```python
from build123d import *

# Parameters (mm, degrees)
SZKIC1_W                       = 90
SZKIC1_H                       = 62
DODANIE_WYCI_GNI_CIE1_DEPTH    = 12
OTW_R_GWINTOWANY_M5X0_81_D     = 4.2
OTW_R_GWINTOWANY_M5X0_81_DEPTH = 14
OTW_R_GWINTOWANY_M5X0_81_TIP   = 1.2618073
OTW_R_GWINTOWANY_M5X0_82_D     = 4.2
OTW_R_GWINTOWANY_M5X0_82_DEPTH = 20
OTW_R_GWINTOWANY_M5X0_82_TIP   = 1.2618073


with BuildPart() as part:
    # Szkic1 → Dodanie-wyciągnięcie1 (new body)
    with BuildSketch(Plane.XY):
        with Locations((73, 300)):
            Rectangle(SZKIC1_W, SZKIC1_H)
    extrude(amount=DODANIE_WYCI_GNI_CIE1_DEPTH)

    # Otwór gwintowany M5x0.81
    with Locations(Plane.XY.offset(12)):
        with Locations((97, 323), (79, 323), (79, 277), (97, 277)):
            Hole(OTW_R_GWINTOWANY_M5X0_81_D / 2, depth=OTW_R_GWINTOWANY_M5X0_81_DEPTH)
            with Locations((0, 0, -(OTW_R_GWINTOWANY_M5X0_81_DEPTH + OTW_R_GWINTOWANY_M5X0_81_TIP / 2))):  # 118° drill point
                Cone(0, OTW_R_GWINTOWANY_M5X0_81_D / 2, OTW_R_GWINTOWANY_M5X0_81_TIP, mode=Mode.SUBTRACT)

    # Otwór gwintowany M5x0.82
    with Locations(Plane.ZY.offset(-28)):
        with Locations((6, 286), (6, 314)):
            Hole(OTW_R_GWINTOWANY_M5X0_82_D / 2, depth=OTW_R_GWINTOWANY_M5X0_82_DEPTH)
            with Locations((0, 0, -(OTW_R_GWINTOWANY_M5X0_82_DEPTH + OTW_R_GWINTOWANY_M5X0_82_TIP / 2))):  # 118° drill point
                Cone(0, OTW_R_GWINTOWANY_M5X0_82_D / 2, OTW_R_GWINTOWANY_M5X0_82_TIP, mode=Mode.SUBTRACT)


solid = part.part
```
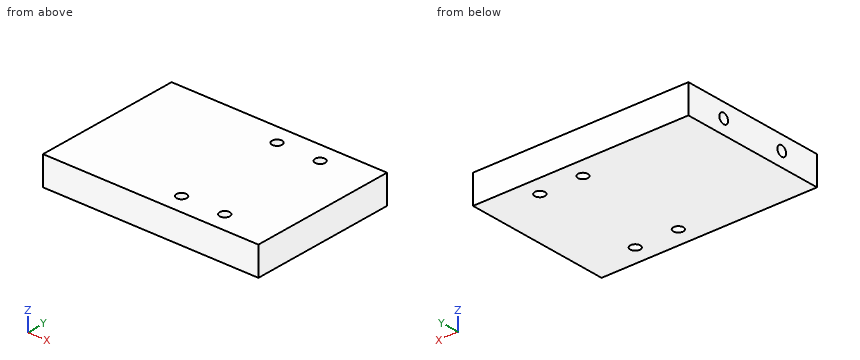
Could you check a few things on this model? Use its own coordinates, in mm. Give positions to 0.01 mm unless a question says otherwise; leave off trailing zeros. Order: outer loops, then holes, each group sorted by start corner. A loop starts at its lowest first (then second) coordinate and runs counter-clockwise, first axis right, second up.
Q1. Suppose I cut it at A-A, the plane x = 79. Write out the boundary of the cut face in (y, z).
Q2. Suppose I cut it at B-B, the plane y = 323. Write out the boundary of the cut face in (x, z), and give its area (3 significant figures).
Q3. Suppose I cut it at C-C, the plane x = 35.5. Write out the boundary of the cut face in (y, z), and give its area (3 significant figures).
Q4. I'm going to push flat-ended pins straight in: P1, Ø3.5, axis at x = 79, y = 277, coming from the +Z side; P2, Ø5, axis at x = 105.5, y = 284, coming from the -Z side; P3, Ø2.5, axis at y = 314, z = 6, coming from the -X side. Where does each tip first touch, or does it pass through?
Q5. If I drill on line 1 along X through (y, z) = (323, 7.5); line 2 along Y through (x, z) = (39, 6); line 3 along Y through (x, z) = (79, 7.25), over which ranges is the centre line in solid material (lowest first)?
Solution:
1. outline: (269, 0) - (274.9, 0) - (274.9, 12) - (269, 12) - close; (279.1, 0) - (320.9, 0) - (320.9, 12) - (279.1, 12) - close; (325.1, 0) - (331, 0) - (331, 12) - (325.1, 12) - close
2. outline: (28, 0) - (76.9, 0) - (76.9, 12) - (28, 12) - close; (81.1, 0) - (94.9, 0) - (94.9, 12) - (81.1, 12) - close; (99.1, 0) - (118, 0) - (118, 12) - (99.1, 12) - close
2. area: 979 mm2
3. outline: (269, 0) - (331, 0) - (331, 12) - (269, 12) - close; hole circle Ø4.2 at (286, 6); hole circle Ø4.2 at (314, 6)
3. area: 716 mm2
4. P1: passes through
4. P2: stops at z = 0
4. P3: stops at x = 48.51
5. line 1: x = 28 to 76.9, 81.1 to 94.9, 99.1 to 118
5. line 2: y = 269 to 283.9, 288.1 to 311.9, 316.1 to 331
5. line 3: y = 269 to 274.9, 279.1 to 320.9, 325.1 to 331
